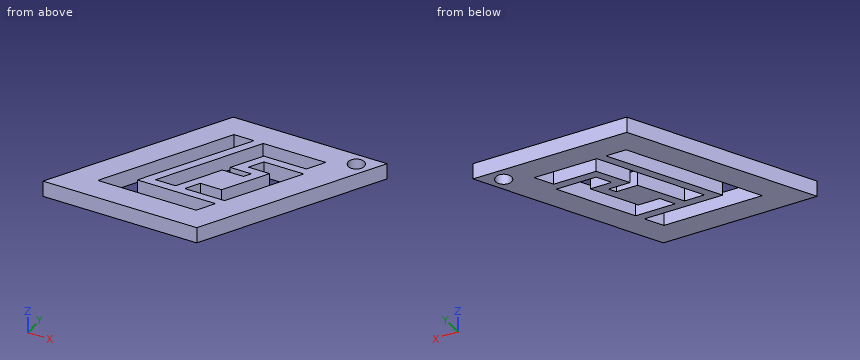
from build123d import *

# Parameters (mm, degrees)
F0_R     = 1
F1_DEPTH = 2


with BuildPart() as f1:
    # F0 (on Top) → F1 (new body)
    with BuildSketch(Plane.XY):
        Polygon((0.368802, -11.361216), (12.564955, 9.76314), (-6.636751, 9.76314), (-18.832904, -11.361216), align=None)
        Polygon((-4.5, -5.196152), (-3.5, -3.464102), (-0.845299, -3.464102), (2.232051, 1.866025), (-0.42265, 1.866025), (0.57735, 3.598076), (5.541452, 3.598076), (0.464102, -5.196152), align=None, mode=Mode.SUBTRACT)
        Polygon((-4.904701, 6.76314), (-2.404701, 6.76314), (-9.886751, -6.196152), (-0.113249, -6.196152), (-1.363249, -8.361216), (-13.636751, -8.361216), align=None, mode=Mode.SUBTRACT)
        Polygon((-5.654701, -5.196152), (-8.154701, -5.196152), (-1.25, 6.76314), (6.559401, 6.76314), (5.309401, 4.598076), (2.654701, 4.598076), (0, 4.598076), (-2.154701, 0.866025), (0.5, 0.866025), (0, 0), (-2.654701, 0), align=None, mode=Mode.SUBTRACT)
        with Locations((9.652769, 8.081789)):
            Circle(F0_R, mode=Mode.SUBTRACT)
    extrude(amount=F1_DEPTH)


solid = f1.part
Here's how the part is built. I have some questions about the finished solid (model axes, mm). Give positions to 0.01 mm unless a question says otherwise; leave off trailing zeros. Write each loop counter-clockwise with the first axis right and the second up, starting at its lowest first coordinate (ties: lowest second). Pieces come first, ordered by that corner, then holes. Notation, with made-up numbers: (-15, -39) -> (5, -39) arc R14 cw to (5, -27) -> close; hole circle Ø6 at (16, 78). An arc over 180 degrees is marked (long way). Use one line per item in the form item = value. Start each with the question number.
1. If I drill on L1, parallel to X at y = 3.5, z = 1.85; L2, parallel to X at y = 1.25, z = 1.35; L3, parallel to Y at x = -5.5, z = 0.9, over which ranges is the centre line in solid material (lowest first)?
2. Will this pin go through, and if not, where does the flat tip stop? pin 1 Ø6 at (x, y) = (6.5, 0.5) entering from -Z.
3. Imagine slicing it at A-A on x = 4.5. List the corners of the cut face in (y, z) for me, plus the area to 3 significant figures.
4. Imagine slicing it at B-B on y = 8.75. List the corners of the cut face in (x, z) for me, plus the area to 3 significant figures.
5. Imagine slicing it at C-C on x = 1. List the corners of the cut face in (y, z) for me.
6. Imagine slicing it at D-D on z = 0.3. State how many separate pieces and enclosed holes the cut face has, plus the area to 3 significant figures.
Entries:
q1.L1 = -10.25 to -6.79, -4.29 to -3.13, -0.63 to 0.52, 5.48 to 8.95
q1.L2 = -11.55 to -8.09, -5.59 to -4.43, -1.93 to 1.88, 4.19 to 7.65
q1.L3 = -11.36 to -8.36, -6.2 to -4.93, -0.6 to 1.4, 5.73 to 9.76
q2.pin_1 = 0
q3.outline = (-4.21, 0) -> (1.79, 0) -> (1.79, 2) -> (-4.21, 2) -> close; (3.6, 0) -> (4.6, 0) -> (4.6, 2) -> (3.6, 2) -> close; (6.76, 0) -> (9.76, 0) -> (9.76, 2) -> (6.76, 2) -> close
q3.area = 20.0 mm²
q4.outline = (-7.22, 0) -> (8.91, 0) -> (8.91, 2) -> (-7.22, 2) -> close; (10.4, 0) -> (11.98, 0) -> (11.98, 2) -> (10.4, 2) -> close
q4.area = 35.4 mm²
q5.outline = (-10.27, 0) -> (-4.27, 0) -> (-4.27, 2) -> (-10.27, 2) -> close; (-0.27, 0) -> (1.87, 0) -> (1.87, 2) -> (-0.27, 2) -> close; (3.6, 0) -> (4.6, 0) -> (4.6, 2) -> (3.6, 2) -> close; (6.76, 0) -> (9.76, 0) -> (9.76, 2) -> (6.76, 2) -> close
q6.separate_pieces = 1
q6.enclosed_holes = 4
q6.area = 270 mm²
